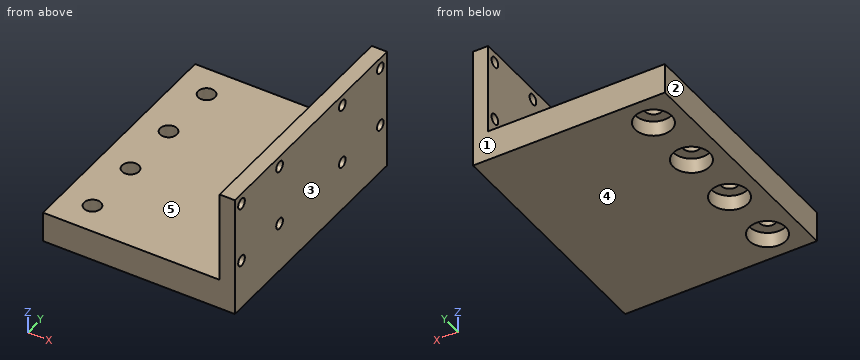
```python
from build123d import *

# Parameters (mm, degrees)
ESQUISSE1_W             = 63
ESQUISSE1_H             = 80
ESQUISSE1_R             = 2.75
BOSS_EXTRU_1_DEPTH      = 10
ESQUISSE2_W             = 5
ESQUISSE2_H             = 80
BOSS_EXTRU_2_DEPTH      = 30
ENL_V_MAT_EXTRU_1_REACH = 95.09
ESQUISSE3_R             = 1.75
ESQUISSE4_R             = 6
ENL_V_MAT_EXTRU_2_DEPTH = 5


with BuildPart() as part:
    # Esquisse1 → Boss.-Extru.1 (new body)
    with BuildSketch(Plane.XY):
        with Locations((-1.896872358, -15.648351648)):
            Rectangle(ESQUISSE1_W, ESQUISSE1_H)
        with Locations((-23.396872358, 14.351648352)):
            Circle(ESQUISSE1_R, mode=Mode.SUBTRACT)
        with Locations((-23.396872358, -5.648351648)):
            Circle(ESQUISSE1_R, mode=Mode.SUBTRACT)
        with Locations((-23.396872358, -25.648351648)):
            Circle(ESQUISSE1_R, mode=Mode.SUBTRACT)
        with Locations((-23.396872358, -45.648351648)):
            Circle(ESQUISSE1_R, mode=Mode.SUBTRACT)
    extrude(amount=BOSS_EXTRU_1_DEPTH)

    # Esquisse2 → Boss.-Extru.2 (add)
    with BuildSketch(Plane(origin=(0, 0, 10), x_dir=(-1, 0, 0), z_dir=(0, 0, -1))):
        with Locations((-27.103127642, -15.648351648)):
            Rectangle(ESQUISSE2_W, ESQUISSE2_H)
    extrude(amount=-BOSS_EXTRU_2_DEPTH)

    # Esquisse3 → Enlèv. mat.-Extru.1 (cut, up to next)
    with BuildSketch(Plane(origin=(29.603127642, 0, 0), x_dir=(0, 0, -1), z_dir=(1, 0, 0)), mode=Mode.PRIVATE) as enl_v_mat_extru_1_sk1:
        with Locations(Location((-36.5, -52.148351648, 0), (0, 0, 90))):
            Circle(ESQUISSE3_R)
    enl_v_mat_extru_1_tool1 = extrude(enl_v_mat_extru_1_sk1.sketch, amount=-ENL_V_MAT_EXTRU_1_REACH, mode=Mode.PRIVATE) & part.part
    # Esquisse3 → Enlèv. mat.-Extru.1 (cut, up to next)
    with BuildSketch(Plane(origin=(29.603127642, 0, 0), x_dir=(0, 0, -1), z_dir=(1, 0, 0)), mode=Mode.PRIVATE) as enl_v_mat_extru_1_sk2:
        with Locations(Location((-36.5, -32.148351648, 0), (0, 0, 90))):
            Circle(ESQUISSE3_R)
    enl_v_mat_extru_1_tool2 = extrude(enl_v_mat_extru_1_sk2.sketch, amount=-ENL_V_MAT_EXTRU_1_REACH, mode=Mode.PRIVATE) & part.part
    # Esquisse3 → Enlèv. mat.-Extru.1 (cut, up to next)
    with BuildSketch(Plane(origin=(29.603127642, 0, 0), x_dir=(0, 0, -1), z_dir=(1, 0, 0)), mode=Mode.PRIVATE) as enl_v_mat_extru_1_sk3:
        with Locations(Location((-16.5, -32.148351648, 0), (0, 0, 90))):
            Circle(ESQUISSE3_R)
    enl_v_mat_extru_1_tool3 = extrude(enl_v_mat_extru_1_sk3.sketch, amount=-ENL_V_MAT_EXTRU_1_REACH, mode=Mode.PRIVATE) & part.part
    # Esquisse3 → Enlèv. mat.-Extru.1 (cut, up to next)
    with BuildSketch(Plane(origin=(29.603127642, 0, 0), x_dir=(0, 0, -1), z_dir=(1, 0, 0)), mode=Mode.PRIVATE) as enl_v_mat_extru_1_sk4:
        with Locations(Location((-16.5, -52.148351648, 0), (0, 0, 90))):
            Circle(ESQUISSE3_R)
    enl_v_mat_extru_1_tool4 = extrude(enl_v_mat_extru_1_sk4.sketch, amount=-ENL_V_MAT_EXTRU_1_REACH, mode=Mode.PRIVATE) & part.part
    # Esquisse3 → Enlèv. mat.-Extru.1 (cut, up to next)
    with BuildSketch(Plane(origin=(29.603127642, 0, 0), x_dir=(0, 0, -1), z_dir=(1, 0, 0)), mode=Mode.PRIVATE) as enl_v_mat_extru_1_sk5:
        with Locations(Location((-36.5, 0.851648352, 0), (0, 0, 90))):
            Circle(ESQUISSE3_R)
    enl_v_mat_extru_1_tool5 = extrude(enl_v_mat_extru_1_sk5.sketch, amount=-ENL_V_MAT_EXTRU_1_REACH, mode=Mode.PRIVATE) & part.part
    # Esquisse3 → Enlèv. mat.-Extru.1 (cut, up to next)
    with BuildSketch(Plane(origin=(29.603127642, 0, 0), x_dir=(0, 0, -1), z_dir=(1, 0, 0)), mode=Mode.PRIVATE) as enl_v_mat_extru_1_sk6:
        with Locations(Location((-36.5, 20.851648352, 0), (0, 0, 90))):
            Circle(ESQUISSE3_R)
    enl_v_mat_extru_1_tool6 = extrude(enl_v_mat_extru_1_sk6.sketch, amount=-ENL_V_MAT_EXTRU_1_REACH, mode=Mode.PRIVATE) & part.part
    # Esquisse3 → Enlèv. mat.-Extru.1 (cut, up to next)
    with BuildSketch(Plane(origin=(29.603127642, 0, 0), x_dir=(0, 0, -1), z_dir=(1, 0, 0)), mode=Mode.PRIVATE) as enl_v_mat_extru_1_sk7:
        with Locations(Location((-16.5, 20.851648352, 0), (0, 0, 90))):
            Circle(ESQUISSE3_R)
    enl_v_mat_extru_1_tool7 = extrude(enl_v_mat_extru_1_sk7.sketch, amount=-ENL_V_MAT_EXTRU_1_REACH, mode=Mode.PRIVATE) & part.part
    # Esquisse3 → Enlèv. mat.-Extru.1 (cut, up to next)
    with BuildSketch(Plane(origin=(29.603127642, 0, 0), x_dir=(0, 0, -1), z_dir=(1, 0, 0)), mode=Mode.PRIVATE) as enl_v_mat_extru_1_sk8:
        with Locations(Location((-16.5, 0.851648352, 0), (0, 0, 90))):
            Circle(ESQUISSE3_R)
    enl_v_mat_extru_1_tool8 = extrude(enl_v_mat_extru_1_sk8.sketch, amount=-ENL_V_MAT_EXTRU_1_REACH, mode=Mode.PRIVATE) & part.part
    add(enl_v_mat_extru_1_tool1.solids().sort_by_distance((29.603128, -52.148352, 36.5))[0], mode=Mode.SUBTRACT)
    add(enl_v_mat_extru_1_tool2.solids().sort_by_distance((29.603128, -32.148352, 36.5))[0], mode=Mode.SUBTRACT)
    add(enl_v_mat_extru_1_tool3.solids().sort_by_distance((29.603128, -32.148352, 16.5))[0], mode=Mode.SUBTRACT)
    add(enl_v_mat_extru_1_tool4.solids().sort_by_distance((29.603128, -52.148352, 16.5))[0], mode=Mode.SUBTRACT)
    add(enl_v_mat_extru_1_tool5.solids().sort_by_distance((29.603128, 0.851648, 36.5))[0], mode=Mode.SUBTRACT)
    add(enl_v_mat_extru_1_tool6.solids().sort_by_distance((29.603128, 20.851648, 36.5))[0], mode=Mode.SUBTRACT)
    add(enl_v_mat_extru_1_tool7.solids().sort_by_distance((29.603128, 20.851648, 16.5))[0], mode=Mode.SUBTRACT)
    add(enl_v_mat_extru_1_tool8.solids().sort_by_distance((29.603128, 0.851648, 16.5))[0], mode=Mode.SUBTRACT)

    # Esquisse4 → Enlèv. mat.-Extru.2 (cut)
    with BuildSketch(Plane(origin=(0, 0, 0), x_dir=(-1, 0, 0), z_dir=(0, 0, -1))):
        with Locations((23.396872358, -45.648351648)):
            Circle(ESQUISSE4_R)
        with Locations((23.396872358, -25.648351648)):
            Circle(ESQUISSE4_R)
        with Locations((23.396872358, -5.648351648)):
            Circle(ESQUISSE4_R)
        with Locations((23.396872358, 14.351648352)):
            Circle(ESQUISSE4_R)
    extrude(amount=-ENL_V_MAT_EXTRU_2_DEPTH, mode=Mode.SUBTRACT)


solid = part.part
```
Work out the finished part from the listing and answer in its coordinate system (mm). Face numbers are marked on the shaded views. A direction names the side the tool comes from. Coordinates: 2 decimals unless noted, no trailing zeros. Write each loop counter-clockwise with the first axis right and the second up, starting at its lowest first coordinate (ties: lowest second). Pieces come first, ordered by that corner, then holes. Notation, with made-up numbers: (55, 21.25) - (97, 21.25) arc R26 ccw to (97, 54.25) - close; hole circle Ø8 at (55.5, 79). An arc over 180 degrees is marked (long way). Answer as a JSON object with one key per item and string values.
Q1. Find section B-B (y = -24). Write down the section's boundary in (x, z), plus the area to 3 significant figures.
Results list:
{"outline": "(-33.4, 0) - (-29.17, 0) - (-29.17, 5) - (-25.6, 5) - (-25.6, 10) - (-33.4, 10) - close; (-21.2, 5) - (-17.63, 5) - (-17.63, 0) - (29.6, 0) - (29.6, 40) - (24.6, 40) - (24.6, 10) - (-21.2, 10) - close", "area": "700 mm^2"}
Q2. Given pin 1 Ø2 at (y, z) = (0.85, 36.5) entering from +X; pin 2 Ø19 at (x, y) = (-23.4, -45.65) entering from +Z; pin 3 Ø6 at (y, z) = (-33, 26) entering from -X; pin 4 Ø9.5 at (x, y) = (-23.4, -5.65) entering from -Z, each flat-ended and moving along its own axis, determine where each tip first touches the part or whether it passes through.
Results list:
{"pin 1": "passes through", "pin 2": "stops at z = 10", "pin 3": "stops at x = 24.6", "pin 4": "stops at z = 5"}
Q3. Find section A-A (z = 36.5). Write down the section's boundary in (x, y).
Results list:
{"outline": "(24.6, -55.65) - (29.6, -55.65) - (29.6, -53.9) - (24.6, -53.9) - close; (24.6, -50.4) - (29.6, -50.4) - (29.6, -33.9) - (24.6, -33.9) - close; (24.6, -30.4) - (29.6, -30.4) - (29.6, -0.9) - (24.6, -0.9) - close; (24.6, 2.6) - (29.6, 2.6) - (29.6, 19.1) - (24.6, 19.1) - close; (24.6, 22.6) - (29.6, 22.6) - (29.6, 24.35) - (24.6, 24.35) - close"}
Q4. Consider L1, parallel to X at y = 11, z = 37; L2, parallel to Z at x = -24.5, y = -28.5; L3, parallel to Z at x = -13, y = 20. Determine where each line is inside the solid, lowest interval first. Write a range as from..to.
Results list:
{"L1": "x = 24.6..29.6", "L2": "z = 5..10", "L3": "z = 0..10"}
Q5. Which of the six approach directions +Z, -Z, +X, -X, +Y, -Y give full straight-line access (tool end or side, diameter ignored) to the marked faces 4 and 5?
Results list:
{"face 4": "-Z, +X, -X, +Y, -Y", "face 5": "+Z, -X, +Y, -Y"}
Q6. Find section D-D (z = 31). Write down the section's boundary in (x, y).
Results list:
{"outline": "(24.6, -55.65) - (29.6, -55.65) - (29.6, 24.35) - (24.6, 24.35) - close"}
Q7. For a pull along X with two mould halves and no side action, classify the marked faces 1, 2 and 3 as pulls with the +X half, pulls with the -X half, needs draft (parallel to the pull), parting line crosses it, or undercut.
Results list:
{"face 1": "needs draft", "face 2": "pulls with the -X half", "face 3": "pulls with the +X half"}
Q8. Find section C-C (x = 20.5). Write down the section's boundary in (y, z).
Results list:
{"outline": "(-55.65, 0) - (24.35, 0) - (24.35, 10) - (-55.65, 10) - close"}
